from build123d import *

# Parameters (mm, degrees)
F0_R     = 31.75
F0_R_2   = 1.651
F1_DEPTH = 10.16
F3_DEPTH = 5.08


with BuildPart() as f1:
    # F0 (on Front) → F1 (new body)
    with BuildSketch(Plane.XZ):
        Circle(F0_R)
        Circle(F0_R_2, mode=Mode.SUBTRACT)
    extrude(amount=F1_DEPTH)

    # F2 (on Front) → F3 (cut)
    with BuildSketch(Plane.XZ):
        with BuildLine():
            Line((0, 13.714062), (4.249023, 20.192205))
            ThreePointArc((4.249023, 20.192205), (-15.124809, 14.036363), (-19.819271, -5.742458))
            Line((-19.819271, -5.742458), (-13.714062, 0))
            ThreePointArc((-13.714062, 0), (-9.697307, 9.697307), (0, 13.714062))
        make_face()
        with BuildLine():
            ThreePointArc((13.714062, 0), (9.697307, -9.697307), (0, -13.714062))
            Line((0, -13.714062), (-2.821576, -20.440598))
            ThreePointArc((-2.821576, -20.440598), (17.210942, -11.382565), (17.705395, 10.59709))
            Line((17.705395, 10.59709), (13.714062, 0))
        make_face()
    extrude(amount=F3_DEPTH, mode=Mode.SUBTRACT)


solid = f1.part
Build history of the part. All positions in model axes, mm. A direction names the side the tool comes from. Coordinates: 2 decimals unless noted, no trailing zeros. Order: outer loops, then holes, each group sorted by start corner. A loop starts at its lowest first (then second) coordinate and runs counter-clockwise, first axis right, second up. Notation, with made-up numbers: M 4,34.5 L 10,34.5 A24 cw 10,73.5 Z; hole C 55.5,-27 d5. An arc over 180 degrees is marked long. One line per question, with ' | ' between items. Start each with the question number.
Q1. Saw through at C-C (y = -7.5). List the corners of the cut face in (x, z).
Q2. Saw through at D-D (x = -5.5). List the corners of the cut face in (y, z).
Q3. Saw through at A-A (x = 11.5). List the corners of the cut face in (y, z).
Q4. Saw through at B-B (z = 4.5). List the corners of the cut face in (x, y).
Q5. Two-plate mould, pull along Z, no slides. Class faces 3 (the face through (-6.883, -5.009, -30.995)), 4 (the face through (-9.803, -2.504, 9.59)), 5 (the face through (-10, -5.08, 10)), 6 (the face through (7, -10.16, 0)): +Z half, -Z half, draft (parallel to the pull), parting line (faces both ways), or undercut.
Q6. Probe L1, parallel to Z at x = 0, y = -5.5; L2, parallel to X at y = -2.25, z = -0.5; L3, parallel to Z at x = -1, y = -9.25. List the from-to ranges inside material, lowest first. Write a range as from..to.
Q7. Flat gauge pins, fed straight in: pin 1 Ø4 at (x, y) = (-17, -1.5) entering from +Z; pin 2 Ø12.5 at (x, z) = (-2.5, 11.5) entering from +Y; pin 3 Ø6 at (x, y) = (5, -2.5) entering from +Z; pin 4 Ø5 at (x, y) = (17.5, -2) entering from -Z. Where does each tip first touch, or does it go through?
Q8. 3-axis set-ups, long thin cutter, end or side, ignore diameter. For faces 1 (the face through (7, 0, 0)), 2 (the face through (-1.39, -2.5, -17.03)): which of +Z, -Z, +X, -X, +Y, -Y reach the whole face in a straight line?
Check values:
1) outline: C 0,0 d63.5; hole C 0,0 d3.3
2) outline: M -10.16,-31.27 L 0,-31.27 L 0,12.56 L -5.08,12.56 L -5.08,19.89 L 0,19.89 L 0,31.27 L -10.16,31.27 Z
3) outline: M -10.16,-29.59 L 0,-29.59 L 0,-17.13 L -5.08,-17.13 L -5.08,-7.47 L 0,-7.47 L 0,29.59 L -10.16,29.59 Z
4) outline: M -31.43,-10.16 L 31.43,-10.16 L 31.43,0 L 20.14,0 L 20.14,-5.08 L 15.41,-5.08 L 15.41,0 L -12.95,0 L -12.95,-5.08 L -20.14,-5.08 L -20.14,0 L -31.43,0 Z
5) face 3: parting line | face 4: undercut | face 5: undercut | face 6: draft
6) L1: z = -31.75..-1.65, 1.65..31.75 | L2: x = -31.75..-20.63, -14.25..-1.57, 1.57..13.7, 20.63..31.75 | L3: z = -31.73..-1.31, 1.31..31.73
7) pin 1: stops at z = 27.98 | pin 2: stops at y = 0 | pin 3: stops at z = 31.69 | pin 4: stops at z = -27.98
8) face 1: +Z, -Z, +X, -X, +Y | face 2: +Y
